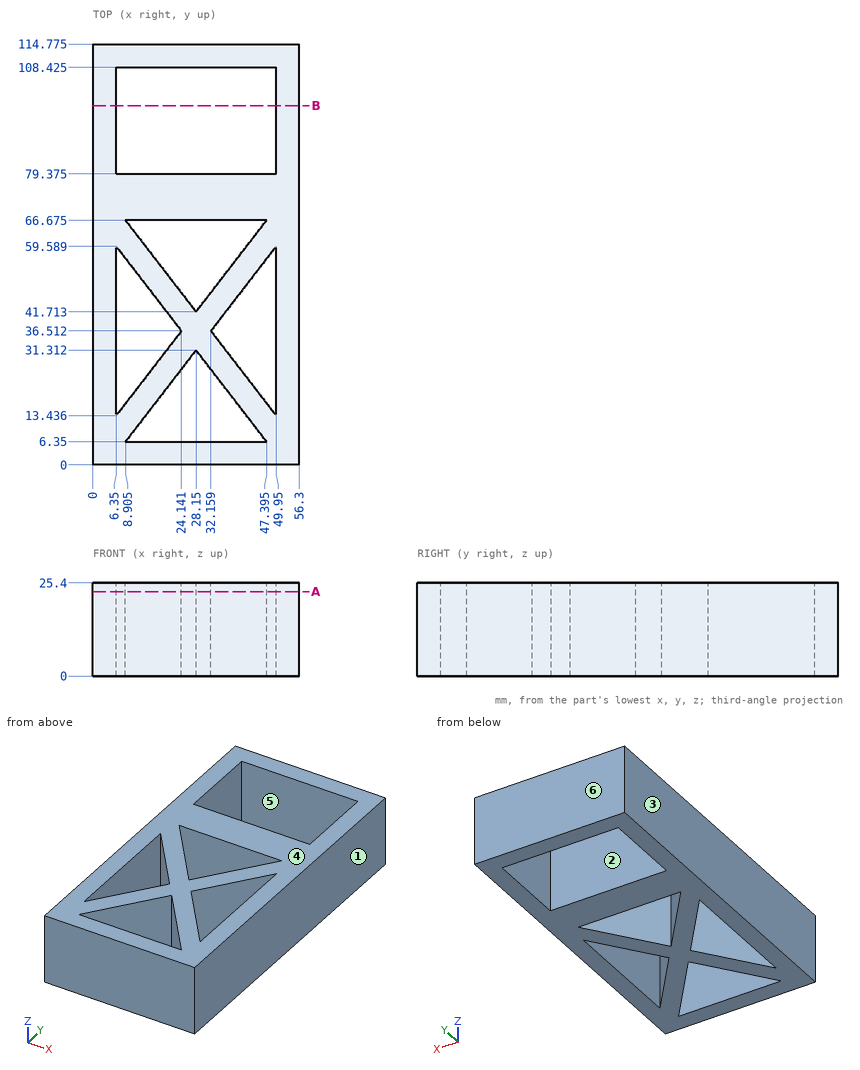
Drawing for the job (mm, zero at the part's lowest x, y, z). A direction names the side the tool comes from. Round coordinates to 2 decimals unless told otherwise and drop trailing zeros. Write each loop counter-clockwise with the first axis right and the second up, starting at its lowest first coordinate (ties: lowest second). Pieces come first, ordered by that corner, then holes.
Item 1: Band-saw the part on A-A on z = 23. Give the number of separate pieces and of enclosed holes in the cut face, then the cut area to 3 significant figures.
Filled in:
separate pieces: 1
enclosed holes: 5
area: 3,410 mm2
Item 2: Mould opens along X. For the marked faces 1, 2, 3 and 4 say: released by +X, released by -X, zero draft, split by the parting line, or undercut.
Filled in:
face 1: released by +X
face 2: undercut
face 3: released by -X
face 4: zero draft
Item 3: Band-saw the part on B-B on y = 98. Write the cut outline in (x, z).
Filled in:
outline: (0, 0) - (6.35, 0) - (6.35, 25.4) - (0, 25.4) - close; (49.95, 0) - (56.3, 0) - (56.3, 25.4) - (49.95, 25.4) - close
Item 4: Tool access for the marked faces 5 and 6: list every direction of +Z, -Z, +X, -X, +Y, -Y with a clear straight run to the whole face (end or side of a thin tool).
Filled in:
face 5: +Z, -Z
face 6: +Z, -Z, +X, -X, +Y
Item 5: Drill centre lines: L1, parallel to X at y = 82, z = 10; L2, parallel to X at y = 41, z = 8.25; L3, parallel to Y at x = 7, z = 11 (1 decimal). Where is each one in solid material? Low to high.
Filled in:
L1: x = 0 to 6.35, 49.95 to 56.3
L2: x = 0 to 6.35, 20.68 to 35.62, 49.95 to 56.3
L3: y = 0 to 14.3, 58.7 to 79.4, 108.4 to 114.8
